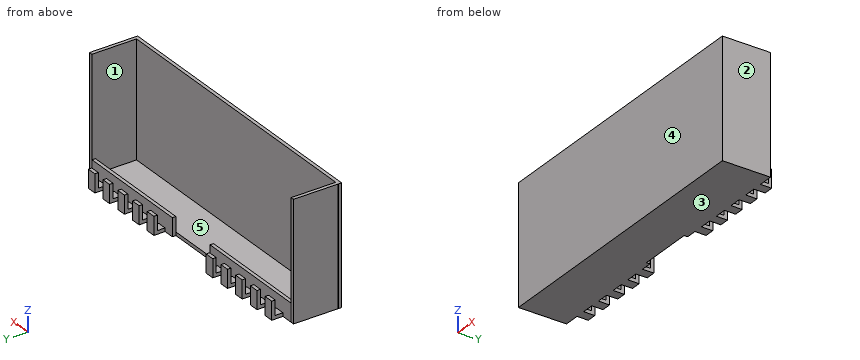
from build123d import *

# Parameters (mm, degrees)
BOSS_EXTRU_1_DEPTH      = 10
ESQUISSE1_W             = 196
ESQUISSE1_H             = 2.35
BOSS_EXTRU_1_2_DEPTH    = 10
ESQUISSE2_W             = 196
ESQUISSE2_H             = 38
BOSS_EXTRU_2_DEPTH      = 2.35
ESQUISSE3_W             = 80.35
ESQUISSE3_H             = 30.346426361
BOSS_EXTRU_4_DEPTH      = 2.35
BOSS_EXTRU_5_DEPTH      = 2.35
BOSS_EXTRU_6_DEPTH      = 68
BOSS_EXTRU_6_DEPTH_BACK = 12.35
ESQUISSE6_W             = 200.815081418
ESQUISSE6_H             = 2.35
ESQUISSE7_W             = 8
ESQUISSE7_H             = 7.65
ENL_V_MAT_EXTRU_1_DEPTH = 13
ESQUISSE9_W             = 37
ESQUISSE9_H             = 12
ENL_V_MAT_EXTRU_2_DEPTH = 13


with BuildPart() as part:
    # Esquisse1 → Boss.-Extru.1 (new body)
    with BuildSketch(Plane.XY):
        Polygon((122.5, 2.35), (122.5, 0), (0, 0), (-73.5, 0), (-73.5, 2.35), align=None)
    extrude(amount=BOSS_EXTRU_1_DEPTH)



with BuildPart() as body_2:
    # Esquisse1 → Boss.-Extru.1 2 (new body)
    with BuildSketch(Plane.XY):
        with Locations((24.5, -6.475)):
            Rectangle(ESQUISSE1_W, ESQUISSE1_H)
    extrude(amount=BOSS_EXTRU_1_2_DEPTH)


with BuildPart() as part_1:
    add(part.part)

    add(body_2.part)  # Boss.-Extru.2 merges body 2
    # Esquisse2 → Boss.-Extru.2 (add)
    with BuildSketch(Plane(origin=(0, 0, 0), x_dir=(-1, 0, 0), z_dir=(0, 0, -1))):
        with Locations((-24.5, -16.65)):
            Rectangle(ESQUISSE2_W, ESQUISSE2_H)
    extrude(amount=BOSS_EXTRU_2_DEPTH)

    # Esquisse3 → Boss.-Extru.4 (add)
    with BuildSketch(Plane.ZY.offset(73.5)):
        with Locations((37.825, -20.47678682)):
            Rectangle(ESQUISSE3_W, ESQUISSE3_H)
    extrude(amount=BOSS_EXTRU_4_DEPTH)

    # Esquisse5 → Boss.-Extru.5 (add)
    with BuildSketch(Plane(origin=(122.5, 0, 0), x_dir=(0, 0, -1), z_dir=(1, 0, 0))):
        Polygon((-78, -5.3), (2.35, -5.303573639), (2.35, -35.65), (-78, -35.65), align=None)
    extrude(amount=BOSS_EXTRU_5_DEPTH)

    # Esquisse6 → Boss.-Extru.6 (add, two sides: drawn at the far end of the back side and taken through both)
    with BuildSketch(Plane.XY.offset(10).offset(-BOSS_EXTRU_6_DEPTH_BACK)):
        with Locations((24.442459291, -36.825)):
            Rectangle(ESQUISSE6_W, ESQUISSE6_H)
    extrude(amount=BOSS_EXTRU_6_DEPTH + BOSS_EXTRU_6_DEPTH_BACK)

    # Esquisse7 → Enlèv. mat.-Extru.1 (cut)
    with BuildSketch(Plane.XY.offset(10)):
        with Locations((-69.5, -1.475)):
            Rectangle(ESQUISSE7_W, ESQUISSE7_H)
        with Locations((-55, -1.475)):
            Rectangle(ESQUISSE7_W, ESQUISSE7_H)
        with Locations((-40.5, -1.475)):
            Rectangle(ESQUISSE7_W, ESQUISSE7_H)
        with Locations((-26, -1.475)):
            Rectangle(ESQUISSE7_W, ESQUISSE7_H)
        with Locations((-11.5, -1.475)):
            Rectangle(ESQUISSE7_W, ESQUISSE7_H)
        with Locations((3, -1.475)):
            Rectangle(ESQUISSE7_W, ESQUISSE7_H)
        with Locations((17.5, -1.475)):
            Rectangle(ESQUISSE7_W, ESQUISSE7_H)
        with Locations((32, -1.475)):
            Rectangle(ESQUISSE7_W, ESQUISSE7_H)
        with Locations((46.5, -1.475)):
            Rectangle(ESQUISSE7_W, ESQUISSE7_H)
        with Locations((61, -1.475)):
            Rectangle(ESQUISSE7_W, ESQUISSE7_H)
        with Locations((75.5, -1.475)):
            Rectangle(ESQUISSE7_W, ESQUISSE7_H)
        with Locations((90, -1.475)):
            Rectangle(ESQUISSE7_W, ESQUISSE7_H)
        with Locations((104.5, -1.475)):
            Rectangle(ESQUISSE7_W, ESQUISSE7_H)
        with Locations((119, -1.475)):
            Rectangle(ESQUISSE7_W, ESQUISSE7_H)
        with Locations((133.5, -1.475)):
            Rectangle(ESQUISSE7_W, ESQUISSE7_H)
        with Locations((148, -1.475)):
            Rectangle(ESQUISSE7_W, ESQUISSE7_H)
        with Locations((162.5, -1.475)):
            Rectangle(ESQUISSE7_W, ESQUISSE7_H)
        with Locations((177, -1.475)):
            Rectangle(ESQUISSE7_W, ESQUISSE7_H)
        with Locations((191.5, -1.475)):
            Rectangle(ESQUISSE7_W, ESQUISSE7_H)
        with Locations((206, -1.475)):
            Rectangle(ESQUISSE7_W, ESQUISSE7_H)
        with Locations((220.5, -1.475)):
            Rectangle(ESQUISSE7_W, ESQUISSE7_H)
        with Locations((235, -1.475)):
            Rectangle(ESQUISSE7_W, ESQUISSE7_H)
        with Locations((249.5, -1.475)):
            Rectangle(ESQUISSE7_W, ESQUISSE7_H)
        with Locations((264, -1.475)):
            Rectangle(ESQUISSE7_W, ESQUISSE7_H)
        with Locations((278.5, -1.475)):
            Rectangle(ESQUISSE7_W, ESQUISSE7_H)
        with Locations((293, -1.475)):
            Rectangle(ESQUISSE7_W, ESQUISSE7_H)
        with Locations((307.5, -1.475)):
            Rectangle(ESQUISSE7_W, ESQUISSE7_H)
        with Locations((322, -1.475)):
            Rectangle(ESQUISSE7_W, ESQUISSE7_H)
        with Locations((336.5, -1.475)):
            Rectangle(ESQUISSE7_W, ESQUISSE7_H)
        with Locations((351, -1.475)):
            Rectangle(ESQUISSE7_W, ESQUISSE7_H)
        with Locations((365.5, -1.475)):
            Rectangle(ESQUISSE7_W, ESQUISSE7_H)
        with Locations((380, -1.475)):
            Rectangle(ESQUISSE7_W, ESQUISSE7_H)
        with Locations((394.5, -1.475)):
            Rectangle(ESQUISSE7_W, ESQUISSE7_H)
        with Locations((409, -1.475)):
            Rectangle(ESQUISSE7_W, ESQUISSE7_H)
        with Locations((423.5, -1.475)):
            Rectangle(ESQUISSE7_W, ESQUISSE7_H)
        with Locations((438, -1.475)):
            Rectangle(ESQUISSE7_W, ESQUISSE7_H)
        with Locations((452.5, -1.475)):
            Rectangle(ESQUISSE7_W, ESQUISSE7_H)
        with Locations((467, -1.475)):
            Rectangle(ESQUISSE7_W, ESQUISSE7_H)
        with Locations((481.5, -1.475)):
            Rectangle(ESQUISSE7_W, ESQUISSE7_H)
        with Locations((496, -1.475)):
            Rectangle(ESQUISSE7_W, ESQUISSE7_H)
        with Locations((510.5, -1.475)):
            Rectangle(ESQUISSE7_W, ESQUISSE7_H)
        with Locations((525, -1.475)):
            Rectangle(ESQUISSE7_W, ESQUISSE7_H)
        with Locations((539.5, -1.475)):
            Rectangle(ESQUISSE7_W, ESQUISSE7_H)
        with Locations((554, -1.475)):
            Rectangle(ESQUISSE7_W, ESQUISSE7_H)
        with Locations((568.5, -1.475)):
            Rectangle(ESQUISSE7_W, ESQUISSE7_H)
        with Locations((583, -1.475)):
            Rectangle(ESQUISSE7_W, ESQUISSE7_H)
        with Locations((597.5, -1.475)):
            Rectangle(ESQUISSE7_W, ESQUISSE7_H)
        with Locations((612, -1.475)):
            Rectangle(ESQUISSE7_W, ESQUISSE7_H)
        with Locations((626.5, -1.475)):
            Rectangle(ESQUISSE7_W, ESQUISSE7_H)
        with Locations((641, -1.475)):
            Rectangle(ESQUISSE7_W, ESQUISSE7_H)
    extrude(amount=-ENL_V_MAT_EXTRU_1_DEPTH, mode=Mode.SUBTRACT)

    # Esquisse9 → Enlèv. mat.-Extru.2 (cut)
    with BuildSketch(Plane.XY.offset(10)):
        with Locations((24.838183524, -1.725435405)):
            Rectangle(ESQUISSE9_W, ESQUISSE9_H)
    extrude(amount=-ENL_V_MAT_EXTRU_2_DEPTH, mode=Mode.SUBTRACT)


solid = part_1.part
CAD build for the part. Positions are in the model's coordinates, mm. Face numbers are marked on the shaded views. A direction names the side the tool comes from. Round coordinates to 2 decimals unless told otherwise and drop trailing zeros. Write each loop counter-clockwise with the first axis right and the second up, starting at its lowest first coordinate (ties: lowest second). Pieces come first, ordered by that corner, then holes. Notation, with made-up numbers: M 47,-12.75 L 76,-12.75 A31 ccw 76,12.25 Z; hole C 39.25,89 d7. An arc over 180 degrees is marked long. Put each result on its own line as item: value. Start each with the question number.
1) Pin check, flat tips, straight feed: pin 1 Ø8 at (x, z) = (40, 17) entering from +Y; pin 2 Ø1 at (y, z) = (-18.5, 50) entering from -X; pin 3 Ø1 at (x, y) = (71.5, -2) entering from +Z. Stop position of each tip, or through.
2) 3-axis set-ups, long thin cutter, end or side, ignore diameter. For the marked faces 4 and 5: which of +Z, -Z, +X, -X, +Y, -Y reach the whole face in a straight line?
3) Saw through at C-C, the plane z = 49. Write the cut outline in (x, y).
4) Saw through at D-D, the plane x = 104. Write the cut outline in (y, z), and give its area (3 significant figures).
5) Drill centre lines: probe 1 along Y at (x, z) = (56.5, 3.5); probe 2 along X at (y, z) = (-34.5, 59.5); probe 3 along Y at (x, z) = (76.5, 4). Where is each one in solid material? Low to high. Write a range as [from, to].
6) Saw through at B-B, the plane y = -23. Write the cut outline in (x, z), and give its area (3 significant figures).
7) Pull direction X, two halves, no side cores. Call the marked faces 1, 2 and 3: pulls with the +X half, pulls with the -X half, needs draft (parallel to the pull), parting line crosses it, or undercut.
8) Saw through at A-A, the plane x = -5. Write the cut outline in (y, z).
Resolved:
1. pin 1: y = -35.65
1. pin 2: x = -75.85
1. pin 3: z = 0
2. face 4: +Z, -Z, +X, -X, -Y
2. face 5: +Z
3. outline: M -75.97,-38 L 124.85,-38 L 124.85,-5.3 L 122.5,-5.3 L 122.5,-35.65 L -73.5,-35.65 L -73.5,-5.3 L -75.85,-5.3 L -75.85,-35.65 L -75.97,-35.65 Z
4. outline: M -38,-2.35 L -5.3,-2.35 L -5.3,10 L -7.65,10 L -7.65,0 L -35.65,0 L -35.65,78 L -38,78 Z
4. area: 284 mm²
5. probe 1: [-38, -35.65], [-7.65, -5.3], [0, 2.35]
5. probe 2: [-75.85, -73.5], [122.5, 124.85]
5. probe 3: [-38, -35.65], [-7.65, -5.3]
6. outline: M -75.85,-2.35 L 124.85,-2.35 L 124.85,78 L 122.5,78 L 122.5,0 L -73.5,0 L -73.5,78 L -75.85,78 Z
6. area: 838 mm²
7. face 1: undercut
7. face 2: pulls with the +X half
7. face 3: needs draft
8. outline: M -38,-2.35 L 2.35,-2.35 L 2.35,10 L 0,10 L 0,0 L -5.3,0 L -5.3,10 L -7.65,10 L -7.65,0 L -35.65,0 L -35.65,78 L -38,78 Z
